Input: part model. Units: mm. Frame: model coordinates. A direction names the side the tool comes from. Coordinates: 2 decimals unless noted, no trailing zeros. Loops run counter-clockwise (first coordinate to the right, second up) from the corner with the lowest first, then second, coordinate; pieces in that order, holes last.
(1) Mould query, pull axis X, two halves, no side actions, for faces 1 (the face through (-2.38, -10.74, 5.92)), 2 (the face through (6.2, -9.3, 0)), 3 (the face through (-4.769, -21.477, 5.916)). Classes: released by +X, released by -X, zero draft, split by the parting line, or undercut.
(2) Section C-C, the plane z = 4. Return loops of the section in (x, y).
(3) Contact query for flat-ended pins moving along their axis: P1, Ø6, axis at x = 7, z = 7, coming from the -Y side; P2, Ø5, axis at x = -13.5, y = -2, coming from the -Z side; P3, Ø4, axis at x = -9.5, z = 4, coming from the -Y side; P4, Ø5, axis at x = 15, z = 3, coming from the -Y side. Output: stop coordinate, or through.
(4) Line query: L1, parallel to Y at x = 0, z = 3.45; L2, parallel to Y at x = -7.5, z = 8.25; L3, parallel to X at y = 19, z = 9.75. Output: solid intervals per line, ascending.
(5) Section A-A, the plane x = 0. Return loops of the section in (y, z), then the cut area to 3 significant figures.
(6) Section D-D, the plane x = -18. Return loops of the section in (y, z), then the cut area to 3 significant figures.
(7) Set-up query: faces 4 (the face through (12.932, -5.362, 9.465)), 5 (the face through (6.2, -9.3, 12)), 6 (the face through (12.932, -5.362, 2.465)). Return all of +Z, -Z, +X, -X, +Y, -Y with unobstructed straight access to the full face (end or side cutting, diameter ignored); none if empty.
```python
from build123d import *

# Parameters (mm, degrees)
F1_R          = 14
F1_R_2        = 11
F2_DEPTH      = 12
F1_R_3        = 22
F1_R_4        = 14.5
F4_R          = 18.25
F4_R_2        = 12.5
F5_DEPTH      = 1
F5_DEPTH_BACK = 1


with BuildPart() as f2:
    # F1 (on Top) → F2 (new body)
    with BuildSketch(Plane.XY):
        Circle(F1_R)
        Circle(F1_R_2, mode=Mode.SUBTRACT)
    extrude(amount=F2_DEPTH)



with BuildPart() as f2b:
    # F1 (on Top) → F2, piece 2 (new body)
    with BuildSketch(Plane.XY):
        Circle(F1_R_3)
        Circle(F1_R_4, mode=Mode.SUBTRACT)
    extrude(amount=F2_DEPTH)


with BuildPart() as f2_1:
    add(f2.part)

    add(f2b.part)  # F5 merges F2b
    # F4 (on mid) → F5 (join, two sides)
    with BuildSketch(Plane.XY.offset(6)) as f5_sk:
        Circle(F4_R)
        Circle(F4_R_2, mode=Mode.SUBTRACT)
    extrude(amount=F5_DEPTH)
    extrude(f5_sk.sketch, amount=-F5_DEPTH_BACK)


solid = f2_1.part
```
Report:
1. face 1: undercut
1. face 2: zero draft
1. face 3: split by the parting line
2. outline: circle Ø44 at (0, 0); circle Ø28 at (0, 0); hole circle Ø29 at (0, 0); hole circle Ø22 at (0, 0)
3. P1: stops at y = -21.63
3. P2: stops at z = 0
3. P3: stops at y = -20.68
3. P4: stops at y = -18.1
4. L1: y = -22 to -14.5, -14 to -11, 11 to 14, 14.5 to 22
4. L2: y = -20.68 to -12.41, -11.82 to -8.05, 8.05 to 11.82, 12.41 to 20.68
4. L3: x = -11.09 to 11.09
5. outline: (-22, 0) - (-14.5, 0) - (-14.5, 5) - (-14, 5) - (-14, 0) - (-11, 0) - (-11, 12) - (-14, 12) - (-14, 7) - (-14.5, 7) - (-14.5, 12) - (-22, 12) - close; (11, 0) - (14, 0) - (14, 5) - (14.5, 5) - (14.5, 0) - (22, 0) - (22, 12) - (14.5, 12) - (14.5, 7) - (14, 7) - (14, 12) - (11, 12) - close
5. area: 254 mm2
6. outline: (-12.65, 0) - (12.65, 0) - (12.65, 12) - (-12.65, 12) - close
6. area: 304 mm2
7. face 4: +Z
7. face 5: +Z, +X, -X, +Y, -Y
7. face 6: -Z
